The model under review builds one solid part; all positions refer to its coordinate system, in mm. Give positions to 0.01 mm unless a question says otherwise; leave off trailing zeros. Loops run counter-clockwise (first coordinate to the right, second up) from the corner with the lowest first, then second, coordinate; pieces in that order, holes last. Notation, with made-up numbers: (-3.5, 16.25) - (37.5, 16.25) arc R6 cw to (37.5, 26.25) - close; hole circle Ø4 at (49, -12.5). An arc over 180 degrees is marked (long way). Answer as a JSON object with one key per item and string values.
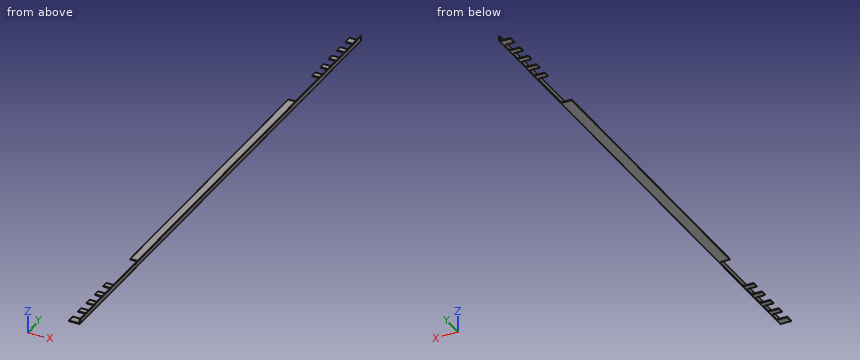
from build123d import *

# Parameters (mm, degrees)
F1_DEPTH = 596.9
F2_R     = 0.76199
F3_W     = 50.8
F3_H     = 101.6
F4_DEPTH = 1.525
F5_W     = 50.8
F5_H     = 22.86
F6_DEPTH = 1.525
F7_R     = 3.175


# Not quite as in the source:
# - a fillet or chamfer is up to 0.001 mm smaller than in the source, because OpenCascade refuses the exact size


with BuildPart() as f1:
    # F0 (on Front) → F1 (new body)
    with BuildSketch(Plane.XZ):
        with BuildLine():
            Line((1.524, 0.762), (1.524, 9.0941772846))
            ThreePointArc((1.524, 9.0941772846), (1.6260886423, 9.4751772846), (1.905, 9.7540886423))
            ThreePointArc((1.905, 9.7540886423), (2.2600354796, 10.6112201124), (1.524, 11.176))
            ThreePointArc((1.524, 11.176), (0.4463692655, 10.7296307345), (0, 9.652))
            Line((0, 9.652), (0, 0.762))
            ThreePointArc((0, 0.762), (-0.2231846327, 0.2231846327), (-0.762, 0))
            Line((-0.762, 0), (-23.876, 0))
            Line((-23.876, 0), (-23.876, -1.524))
            Line((-23.876, -1.524), (-0.762, -1.524))
            ThreePointArc((-0.762, -1.524), (0.8544461018, -0.8544461018), (1.524, 0.762))
        make_face()
    extrude(amount=F1_DEPTH)

    # F2 (radius 0.762 in the source; OpenCascade refuses exactly that, so slightly less here)
    f2_edges = [f1.edges().sort_by_distance(p)[0] for p in [
        (-23.876, -298.45, 0),
        (-23.876, -298.45, -1.524),
    ]]
    fillet(f2_edges, radius=F2_R)

    # F3 (on Top) → F4 (cut, through all)
    with BuildSketch(Plane.XY):
        with Locations((-26.924, -387.35)):
            Rectangle(F3_W, F3_H)
    extrude(amount=-F4_DEPTH, mode=Mode.SUBTRACT)

    # F5 (on Top) → F6 (cut, through all)
    with BuildSketch(Plane.XY):
        with Locations((-26.924, -462.28)):
            Rectangle(F5_W, F5_H)
        with Locations((-26.924, -497.84)):
            Rectangle(F5_W, F5_H)
        with Locations((-26.924, -533.4)):
            Rectangle(F5_W, F5_H)
        with Locations((-26.924, -568.96)):
            Rectangle(F5_W, F5_H)
    extrude(amount=-F6_DEPTH, mode=Mode.SUBTRACT)

    # F7
    f7_edges = [f1.edges().sort_by_distance(p)[0] for p in [
        (-1.524, -336.55, -0.762),
        (-1.524, -438.15, -0.762),
        (-1.524, -450.85, -0.762),
        (-1.524, -473.71, -0.762),
        (-1.524, -509.27, -0.762),
        (-1.524, -544.83, -0.762),
        (-1.524, -580.39, -0.762),
        (-1.524, -486.41, -0.762),
        (-1.524, -521.97, -0.762),
        (-1.524, -557.53, -0.762),
    ]]
    fillet(f7_edges, radius=F7_R)

    # F8: F1 across plane


with BuildPart() as f1_1:
    add(f1.part)
    add(f1.part.mirror(Plane.XZ))


solid = f1_1.part
Q1. Consider section B-B, the plane x = -10.75. State how many separate pieces and enclosed holes the cut face has, plus the area to 3 significant figures.
Results:
{"separate pieces": "11", "enclosed holes": "0", "area": "1,230 mm^2"}
Q2. Consider section C-C, the plane z = 5. State the section outline as (x, y) points.
Results:
{"outline": "(0, -596.9) - (1.52, -596.9) - (1.52, 596.9) - (0, 596.9) - close"}
Q3. Clearance check with flat-ended pins moving along their axes: pin 1 Ø4 at (y, z) = (-382, 6.5) entering from -X; pin 2 Ø10 at (x, y) = (-19, -122) entering from +Z; pin 3 Ø0.5 at (y, z) = (-393.5, -1) entering from -X. State where each tip first meets the part, or that it passes through.
Results:
{"pin 1": "stops at x = 0", "pin 2": "stops at z = 0", "pin 3": "stops at x = -1.52"}
Q4. Consider section A-A, the plane y = -359. State the section outline as (x, z) points (3 decimals), plus the area to 3 significant figures.
Results:
{"outline": "(-1.524, -1.524) - (-0.762, -1.524) arc R2.286 ccw to (1.524, 0.762) - (1.524, 9.094) arc R0.762 cw to (1.905, 9.754) arc R0.762 ccw to (1.524, 11.176) arc R1.524 ccw to (0, 9.652) - (0, 0.762) arc R0.762 cw to (-0.762, 0) - (-1.524, 0) - close", "area": "21.1 mm^2"}
Q5. To check wall thickness, follow probe 1 along X at (y, z) = (-75, 10.25); probe 2 along X at (y, z) = (350, 9); probe 3 along Z at (x, y) = (-10, 33). State the ranges of each line that lie inside material, in increasing order. Write a range as [from, to].
Results:
{"probe 1": "x = [0.12, 2.27]", "probe 2": "x = [0, 1.52]", "probe 3": "z = [-1.52, 0]"}
